Work out the finished part from the listing and answer in its coordinate system (mm). Give positions to 0.01 mm unless a question says otherwise; leave off trailing zeros. Order: outer loops, then holes, each group sorted by start corner. A loop starts at its lowest first (then second) coordinate and runs counter-clockwise, first axis right, second up. Notation, with made-up numbers: (44, 43) - (64, 43) arc R20 ccw to (64, 67) - close; hole circle Ø6 at (53, -33.5). An arc over 180 degrees is marked (long way). Put each result on its own line as item: value.
Autodesk Inventor part; units mm, degrees
ref_plane "YZ Plane" through (0, 0, 0) normal (1, 0, 0) x (0, 1, 0)
ref_plane "XZ Plane" through (0, 0, 0) normal (0, 1, 0) x (-1, 0, 0)
ref_plane "XY Plane" through (0, 0, 0) normal (0, 0, 1) x (1, 0, 0)
sketch "Sketch2" plane through (0, 0, 0) normal (0, 1, 0) x (-1, 0, 0)
  line L0 (0, 0) -> (6, 0)
  line L1 (6, 0) -> (0, 0)
  line L2 (0, -10) -> (6, -10)
  line L3 (3, 0) -> (8, 0)
  line L4 (8, -10) -> (3, -10)
  line L5 (3, -10) -> (-2, -10)
  line L6 (-2, 0) -> (3, 0)
  circle A0 centre (3, 0) radius 1.5
  circle A1 centre (3, 0) radius 3
  circle A2 centre (3, -10) radius 1.5
  circle A3 centre (3, -10) radius 3
  line L7 (0, 0) -> (0, -10)
  line L8 (6, 0) -> (6, -10)
  dimension "d24" = 10
  dimension "d30" = 5
  dimension "d31" = 5
  dimension "d32" = 3
  dimension "d33" = 6
  dimension "d34" = 3
  dimension "d35" = 6
extrude "Extrusion4" add sketch "Sketch2" along normal blind 1 contours A0 L0 A1 | L0 A1 A0 | L8 A3 L7 A1 | A3 L2 A2 | L2 A2 A3
thread "Thread1"
thread "Thread2"
properties part number "linkToActuator4"
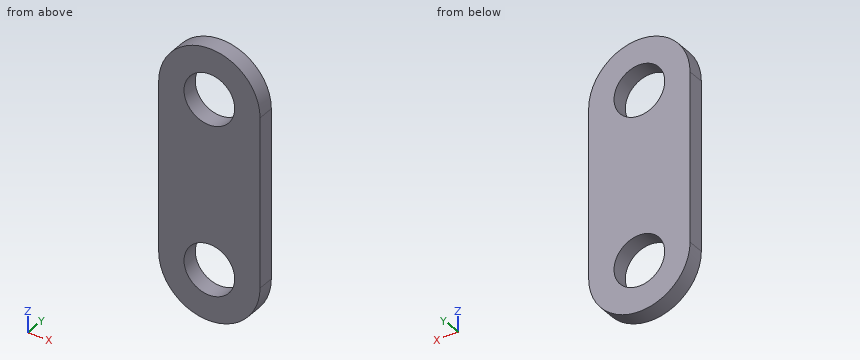
(1) Straight lines are drawn through the part: line 1 (Z direction, x = -3, y = 0.3); line 2 (X direction, y = 0.3, z = 0); line 3 (Z direction, x = -3.85, y = 0.8). For each, find the intervals that lie inside material, in ascending order.
Geometry check:
line 1: z = -13 to -11.5, -8.5 to -1.5, 1.5 to 3
line 2: x = -6 to -4.5, -1.5 to 0
line 3: z = -12.88 to -11.24, -8.76 to -1.24, 1.24 to 2.88
(2) Section D-D, the plane x = -1.95 is taken. Write down the section's boundary in (y, z), then the cut area to 3 significant figures.
Geometry check:
outline: (0, -12.81) - (1, -12.81) - (1, -11.07) - (0, -11.07) - close; (0, -8.93) - (1, -8.93) - (1, -1.07) - (0, -1.07) - close; (0, 1.07) - (1, 1.07) - (1, 2.81) - (0, 2.81) - close
area: 11.3 mm²
(3) Section A-A, the plane x = -3 is taken. Write down the section's boundary in (y, z).
Geometry check:
outline: (0, -13) - (1, -13) - (1, -11.5) - (0, -11.5) - close; (0, -8.5) - (1, -8.5) - (1, -1.5) - (0, -1.5) - close; (0, 1.5) - (1, 1.5) - (1, 3) - (0, 3) - close
(4) Section B-B, the plane y = 0.8 is taken. Write down the section's boundary in (x, z).
Geometry check:
outline: (-6, -10) arc R3 ccw to (0, -10) - (0, 0) arc R3 ccw to (-6, 0) - close; hole circle Ø3 at (-3, -10); hole circle Ø3 at (-3, 0)
(5) Section C-C, the plane x = -5.4 is taken. Write down the section's boundary in (y, z).
Geometry check:
outline: (0, -11.8) - (1, -11.8) - (1, 1.8) - (0, 1.8) - close
